Part model, mm, in its own coordinate system. A direction names the side the tool comes from. Round coordinates to 2 decimals unless told otherwise and drop trailing zeros. Write each loop counter-clockwise with the first axis right and the second up, starting at its lowest first coordinate (ties: lowest second). Pieces come first, ordered by that corner, then holes.
```python
from build123d import *

# Parameters (mm, degrees)
SKETCH_1_W             = 45
SKETCH_1_H             = 10
EXTRUDE_1_DEPTH        = 2
SKETCH_2_W             = 45
SKETCH_2_H             = 23
EXTRUDE_2_DEPTH        = 2
SKETCH_4_W             = 45
SKETCH_4_H             = 2
EXTRUDE_3_DEPTH        = 10
HOLE_START             = -18
HOLE_WIZARD_M3_9_DEPTH = 2
HOLE_WIZARD_M3_1_DEPTH = 2
SKETCH_9_W             = 8
SKETCH_9_H             = 2
CUT_EXTRUDE_1_DEPTH    = 30.904013109
FILLET_2_R             = 3
SKETCH_10_W            = 45
SKETCH_10_H            = 7
CUT_EXTRUDE_2_DEPTH    = 10
SKETCH_11_W            = 45
SKETCH_11_H            = 16
EXTRUDE_4_DEPTH        = 2
HOLE_WIZARD_M3_5_DEPTH = 2
SKETCH_14_W            = 12.097238659
SKETCH_14_H            = 15.369634007
CUT_EXTRUDE_3_DEPTH    = 29.324018077
SKETCH_15_W            = 45
SKETCH_15_H            = 3
CUT_EXTRUDE_4_DEPTH    = 10
FILLET_8_R             = 5
FILLET_9_R             = 1
CUT_EXTRUDE_6_REACH    = 31.904
SKETCH_21_W            = 8
SKETCH_21_H            = 13
FILLET_10_R            = 1
CUT_EXTRUDE_8_REACH    = 31.904
SKETCH_23_W            = 44.634703277
SKETCH_23_H            = 2.5


# Read off the part's stored shape, not the designer's step: M3 间隙槽口9, M3 间隙槽口1, M3 间隙槽口5
with BuildPart() as part:
    # 草图1 → 凸台-拉伸1 (new body)
    with BuildSketch(Plane.XY):
        Rectangle(SKETCH_1_W, SKETCH_1_H)
    extrude(amount=EXTRUDE_1_DEPTH)

    # 草图2 → 凸台-拉伸2 (add)
    with BuildSketch(Plane.XY):
        with Locations((0, -6.5)):
            Rectangle(SKETCH_2_W, SKETCH_2_H)
    extrude(amount=EXTRUDE_2_DEPTH)

    # 草图4 → 凸台-拉伸3 (add)
    with BuildSketch(Plane.XY):
        with Locations((0, -17)):
            Rectangle(SKETCH_4_W, SKETCH_4_H)
    extrude(amount=EXTRUDE_3_DEPTH)

    # M3 间隙槽口9 outline → M3 间隙槽口9 (cut)
    with BuildSketch(Plane(origin=(0, 0, 0), x_dir=(1, 0, 0), z_dir=(0, 1, 0)).offset(HOLE_START)):
        with BuildLine():
            Line((-2.3, -7.7), (2.3, -7.7))
            ThreePointArc((2.3, -7.7), (4, -6), (2.3, -4.3))
            Line((2.3, -4.3), (-2.3, -4.3))
            ThreePointArc((-2.3, -4.3), (-4, -6), (-2.3, -7.7))
        make_face()
    extrude(amount=HOLE_WIZARD_M3_9_DEPTH, mode=Mode.SUBTRACT)

    # M3 间隙槽口1 outline → M3 间隙槽口1 (cut)
    with BuildSketch(Plane.XY):
        with BuildLine():
            ThreePointArc((20.2, 1.3), (18.5, 3), (16.8, 1.3))
            Line((16.8, 1.3), (16.8, -13.3))
            ThreePointArc((16.8, -13.3), (18.5, -15), (20.2, -13.3))
            Line((20.2, -13.3), (20.2, 1.3))
        make_face()
        with BuildLine():
            ThreePointArc((-16.8, 1.3), (-18.5, 3), (-20.2, 1.3))
            Line((-20.2, 1.3), (-20.2, -13.3))
            ThreePointArc((-20.2, -13.3), (-18.5, -15), (-16.8, -13.3))
            Line((-16.8, -13.3), (-16.8, 1.3))
        make_face()
    extrude(amount=HOLE_WIZARD_M3_1_DEPTH, mode=Mode.SUBTRACT)

    # 草图9 → 切除-拉伸1 (cut, through all)
    with BuildSketch(Plane.XY.offset(2)):
        with Locations((-18.5, -17)):
            Rectangle(SKETCH_9_W, SKETCH_9_H)
        with Locations((18.5, -17)):
            Rectangle(SKETCH_9_W, SKETCH_9_H)
    extrude(amount=CUT_EXTRUDE_1_DEPTH, mode=Mode.SUBTRACT)

    # 圆角2
    fillet_2_edges = [part.edges().sort_by_distance(p)[0] for p in [
        (-14.5, -17, 2),
        (14.5, -17, 2),
    ]]
    fillet(fillet_2_edges, radius=FILLET_2_R)

    # 草图10 → 切除-拉伸2 (cut)
    with BuildSketch(Plane.XY.offset(2)):
        with Locations((0, 1.5)):
            Rectangle(SKETCH_10_W, SKETCH_10_H)
    extrude(amount=-CUT_EXTRUDE_2_DEPTH, mode=Mode.SUBTRACT)

    # 草图11 → 凸台-拉伸4 (add)
    with BuildSketch(Plane.XY.offset(2)):
        with Locations((0, -10)):
            Rectangle(SKETCH_11_W, SKETCH_11_H)
    extrude(amount=-EXTRUDE_4_DEPTH)

    # M3 间隙槽口5 outline → M3 间隙槽口5 (cut)
    with BuildSketch(Plane.XY):
        with BuildLine():
            Line((16.8, -10.2), (16.8, -11.8))
            ThreePointArc((16.8, -11.8), (18.5, -13.5), (20.2, -11.8))
            Line((20.2, -11.8), (20.2, -10.2))
            ThreePointArc((20.2, -10.2), (18.5, -8.5), (16.8, -10.2))
        make_face()
        with BuildLine():
            Line((-20.2, -10.2), (-20.2, -11.8))
            ThreePointArc((-20.2, -11.8), (-18.5, -13.5), (-16.8, -11.8))
            Line((-16.8, -11.8), (-16.8, -10.2))
            ThreePointArc((-16.8, -10.2), (-18.5, -8.5), (-20.2, -10.2))
        make_face()
    extrude(amount=HOLE_WIZARD_M3_5_DEPTH, mode=Mode.SUBTRACT)

    # 草图14 → 切除-拉伸3 (cut, through all)
    with BuildSketch(Plane(origin=(0, -16, 0), x_dir=(1, 0, 0), z_dir=(0, 1, 0))):
        with Locations((-14.04861933, -9.684817004)):
            Rectangle(SKETCH_14_W, SKETCH_14_H)
        with Locations((14.04861933, -9.684817004)):
            Rectangle(SKETCH_14_W, SKETCH_14_H)
    extrude(amount=-CUT_EXTRUDE_3_DEPTH, mode=Mode.SUBTRACT)

    # 草图15 → 切除-拉伸4 (cut)
    with BuildSketch(Plane.XY.offset(2)):
        with Locations((0, -3.5)):
            Rectangle(SKETCH_15_W, SKETCH_15_H)
    extrude(amount=-CUT_EXTRUDE_4_DEPTH, mode=Mode.SUBTRACT)

    # 圆角8
    fillet_8_edges = [part.edges().sort_by_distance(p)[0] for p in [
        (8, -17, 10),
        (-8, -17, 10),
    ]]
    fillet(fillet_8_edges, radius=FILLET_8_R)

    # 圆角9
    fillet_9_edges = [part.edges().sort_by_distance(p)[0] for p in [
        (0, -16, 2),
    ]]
    fillet(fillet_9_edges, radius=FILLET_9_R)

    # 草图21 → 切除-拉伸6 (cut, up to next)
    with BuildSketch(Plane.XY.offset(2), mode=Mode.PRIVATE) as cut_extrude_6_sk1:
        with Locations((-18.5, -11.5)):
            Rectangle(SKETCH_21_W, SKETCH_21_H)
    cut_extrude_6_tool1 = extrude(cut_extrude_6_sk1.sketch, amount=-CUT_EXTRUDE_6_REACH, mode=Mode.PRIVATE) & part.part
    add(cut_extrude_6_tool1.solids().sort_by_distance((-18.5, -11.5, 2))[0], mode=Mode.SUBTRACT)

    # 圆角10
    fillet_10_edges = [part.edges().sort_by_distance(p)[0] for p in [
        (22.5, -18, 1),
        (22.5, -5, 1),
        (-14.5, -5, 1),
        (-14.5, -18, 1),
    ]]
    fillet(fillet_10_edges, radius=FILLET_10_R)

    # 草图23 → 切除-拉伸8 (cut, up to next)
    with BuildSketch(Plane.XY.offset(2), mode=Mode.PRIVATE) as cut_extrude_8_sk1:
        with Locations((0.182648362, -6.25)):
            Rectangle(SKETCH_23_W, SKETCH_23_H)
    cut_extrude_8_tool1 = extrude(cut_extrude_8_sk1.sketch, amount=-CUT_EXTRUDE_8_REACH, mode=Mode.PRIVATE) & part.part
    add(cut_extrude_8_tool1.solids().sort_by_distance((0.182648, -6.25, 2))[0], mode=Mode.SUBTRACT)


solid = part.part
```
Q1. Mould opens along X. For faces 1 (the flat face through (4, -13, 2)), 2 (the flat face through (0, -17, 4.3)), 3 (the cylindrical face through (-4, -17, 6)), 4 (the cylindrical face through (-7, -17, 8)) say: +X half, -X half, draft (parallel to the pull), parting line (faces both ways), or undercut.
Values follow:
face 1: draft
face 2: undercut
face 3: undercut
face 4: -X half
Q2. Wall check: L1, parallel to Z at x = -2, y = -16.75; L2, parallel to Y at x = -1, z = 9.25; L3, parallel to Z at x = -9, y = -12.5. Give the ranges that are in metal, low to high.
Values follow:
L1: z = 0 to 4.3, 7.7 to 10
L2: y = -18 to -16
L3: z = 0 to 2
Q3. Cut at B-B on x = 18.5. Write the cut outline in (y, z), plus the area to 3 significant figures.
Values follow:
outline: (-18, 0) - (-13.5, 0) - (-13.5, 2) - (-18, 2) - close; (-8.5, 0) - (-7.5, 0) - (-7.5, 2) - (-8.5, 2) - close
area: 11.0 mm2
Q4. Drop flat-ended pins along their axis: pin 1 (3.5 mm diameter, centred on y = -16, z = 4, fed in from -X); pin 2 (2.5 mm diameter, centred on y = -16.5, z = 4, fed in from +X); pin 3 (5.5 mm diameter, centred on x = 3.5, z = 6.5, fed in from +Y). Give the stop position or say it passes through.
Values follow:
pin 1: stops at x = -8
pin 2: stops at x = 8
pin 3: stops at y = -16
Q5. Cut at C-C on x = 6. Write the cut outline in (y, z).
Values follow:
outline: (-18, 0) - (-7.5, 0) - (-7.5, 2) - (-15, 2) arc R1 cw to (-16, 3) - (-16, 9) - (-18, 9) - close
Q6. Cut at D-D on y = -15.5. Write the cut outline in (x, z).
Values follow:
outline: (-14.5, 0) - (22.5, 0) - (22.5, 2) - (8, 2) - (8, 2.13) - (-8, 2.13) - (-8, 2) - (-14.5, 2) - close
Q7. Which spindle directions (+Z, -Z, +X, -X, +Y, -Y) get a long thin tool onto all of the face, cutting with end or side? Do faces 5 (the cylindrical face through (18.5, -8.5, 1)), 6 (the flat face through (0, -16, 8)), 7 (the cylindrical face through (4, -17, 6)), 8 (the flat face through (4, -13, 0)), 9 (the flat face through (8, -17, 4)). Say none if no direction does.
Values follow:
face 5: +Z, -Z
face 6: +Z, +X, -X, +Y
face 7: +Y, -Y
face 8: -Z, +X, -X, +Y, -Y
face 9: +Z, +X, +Y, -Y
Q8. Cut at A-A on y = -11. Write the cut outline in (x, z).
Values follow:
outline: (-14.5, 0) - (16.8, 0) - (16.8, 2) - (-14.5, 2) - close; (20.2, 0) - (22.5, 0) - (22.5, 2) - (20.2, 2) - close
